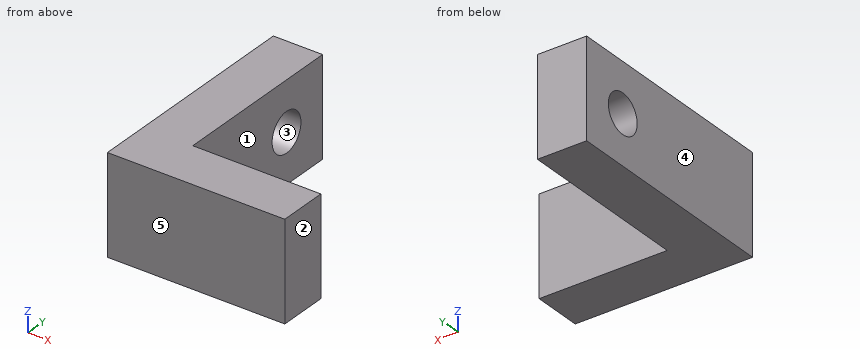
from build123d import *

# Parameters (mm, degrees)
SALIENTE_EXTRUIR1_DEPTH = 5
CROQUIS2_R              = 2
CORTAR_EXTRUIR1_DEPTH   = 27.888659319


with BuildPart() as part:
    # Croquis1 → Saliente-Extruir1 (new, symmetric)
    with BuildSketch(Plane.XY):
        Polygon((0, 0), (0, 23), (5, 23), (5, 5), (18, 5), (18, 0), align=None)
    extrude(amount=SALIENTE_EXTRUIR1_DEPTH, both=True)

    # Croquis2 → Cortar-Extruir1 (cut, through all)
    with BuildSketch(Plane(origin=(5, 0, 0), x_dir=(0, 0, -1), z_dir=(1, 0, 0))):
        with Locations((0, 18)):
            Circle(CROQUIS2_R)
    extrude(amount=-CORTAR_EXTRUIR1_DEPTH, mode=Mode.SUBTRACT)


solid = part.part
Model file for the job. Use its own axes, mm. Face numbers are marked on the shaded views. A direction names the side the tool comes from. Round coordinates to 2 decimals unless told otherwise and drop trailing zeros. Loops run counter-clockwise (first coordinate to the right, second up) from the corner with the lowest first, then second, coordinate; pieces in that order, holes last. Notation, with made-up numbers: (-21, 13) - (-16, 13) arc R8 cw to (-16, 24) - close; hole circle Ø4 at (10, 4.25). An arc over 180 degrees is marked (long way). Write each question's results on one line, items separated by ' | '.
(1) Saw through at B-B, the plane y = 18. List the corners of the cut face in (x, z).
Answer below:
outline: (0, -5) - (5, -5) - (5, -2) - (0, -2) - close; (0, 2) - (5, 2) - (5, 5) - (0, 5) - close
(2) Saw through at D-D, the plane y = 9. List the corners of the cut face in (x, z).
Answer below:
outline: (0, -5) - (5, -5) - (5, 5) - (0, 5) - close
(3) Saw through at A-A, the plane z = 0. List the corners of the cut face in (x, y), then the cut area to 3 significant figures.
Answer below:
outline: (0, 0) - (18, 0) - (18, 5) - (5, 5) - (5, 16) - (0, 16) - close; (0, 20) - (5, 20) - (5, 23) - (0, 23) - close | area: 160 mm^2
(4) Wall check: L1, parallel to Y at x = 3.4, z = 0; L2, parallel to Y at x = 16.5, z = 3.5. Give the ranges that are in metal, low to high.
Answer below:
L1: y = 0 to 16, 20 to 23 | L2: y = 0 to 5
(5) Saw through at C-C, the plane x = 2.75. List the corners of the cut face in (y, z).
Answer below:
outline: (0, -5) - (23, -5) - (23, 5) - (0, 5) - close; hole circle Ø4 at (18, 0)
(6) Mould opens along Y. For the marked faces 3, 4 and 5 say: released by +Y, released by -Y, zero draft, split by the parting line, or undercut.
Answer below:
face 3: undercut | face 4: zero draft | face 5: released by -Y
(7) 3-axis set-ups, long thin cutter, end or side, ignore diameter. For the marked faces 1 and 2: which of +Z, -Z, +X, -X, +Y, -Y reach the whole face in a straight line?
Answer below:
face 1: +Z, -Z, +X, +Y | face 2: +Z, -Z, +X, +Y, -Y
(8) Pin check, flat tips, straight feed: pin 1 (4.5 mm diameter, centred on y = 18, z = 0, fed in from +X); pin 2 (5 mm diameter, centred on x = 14, z = -1, fed in from +Y). Stop position of each tip, or through.
Answer below:
pin 1: stops at x = 5 | pin 2: stops at y = 5
